```python
from build123d import *

# Parameters (mm, degrees)
ESQUISSE1_R               = 1.25
ESQUISSE1_R_2             = 1.5
ESQUISSE1_W               = 23
ESQUISSE1_H               = 12.5
ESQUISSE1_W_2             = 13
ESQUISSE1_H_2             = 3
ESQUISSE1_W_3             = 3
ESQUISSE1_H_3             = 6
ESQUISSE1_W_4             = 5
ESQUISSE1_W_5             = 5.008466432
ESQUISSE1_W_6             = 3.2
ESQUISSE1_H_4             = 2
T_LE_DE_BASE_PLI_E1_DEPTH = 3
ESQUISSE2_R               = 1.5
ENL_V_MAT_EXTRU_1_DEPTH   = 10


# Sheet-metal steps are written as plain solids
with BuildPart() as part:
    # Esquisse1 → Tôle de base pliée1 (new body)
    with BuildSketch(Plane.XY):
        with BuildLine():
            Line((0, 42.516223037), (0, 2))
            ThreePointArc((0, 2), (0.585786438, 0.585786438), (2, 0))
            Line((2, 0), (58, 0))
            ThreePointArc((58, 0), (59.414213562, 0.585786438), (60, 2))
            Line((60, 2), (60, 40.598160001))
            ThreePointArc((60, 40.598160001), (59.938461819, 41.090466587), (59.757634225, 41.552477522))
            Line((59.757634225, 41.552477522), (54.409971269, 51.401647463))
            ThreePointArc((54.409971269, 51.401647463), (53.538493891, 52.240295654), (52.342948156, 52.423254667))
            Line((52.342948156, 52.423254667), (1.690611112, 44.492147761))
            ThreePointArc((1.690611112, 44.492147761), (0.480332639, 43.816458059), (0, 42.516223037))
        make_face()
        with Locations((51.745273693, 48.75)):
            Circle(ESQUISSE1_R, mode=Mode.SUBTRACT)
        with Locations((20.7, 41.7)):
            Circle(ESQUISSE1_R_2, mode=Mode.SUBTRACT)
        with Locations((4.5, 11)):
            Circle(ESQUISSE1_R_2, mode=Mode.SUBTRACT)
        with Locations((55.5, 11)):
            Circle(ESQUISSE1_R_2, mode=Mode.SUBTRACT)
        with Locations((20.5, 31.75)):
            Rectangle(ESQUISSE1_W, ESQUISSE1_H, mode=Mode.SUBTRACT)
        with Locations((46.2, 6)):
            Rectangle(ESQUISSE1_W_2, ESQUISSE1_H_2, mode=Mode.SUBTRACT)
        with Locations((55.7, 4.5)):
            Rectangle(ESQUISSE1_W_3, ESQUISSE1_H_3, mode=Mode.SUBTRACT)
        with Locations((55.7, 17.5)):
            Rectangle(ESQUISSE1_W_3, ESQUISSE1_H_3, mode=Mode.SUBTRACT)
        with Locations((17.808466432, 6)):
            Rectangle(ESQUISSE1_W_4, ESQUISSE1_H_2, mode=Mode.SUBTRACT)
        with Locations((9.804233216, 6)):
            Rectangle(ESQUISSE1_W_5, ESQUISSE1_H_2, mode=Mode.SUBTRACT)
        with Locations((4.3, 6)):
            Rectangle(ESQUISSE1_W_3, ESQUISSE1_H_2, mode=Mode.SUBTRACT)
        with Locations((4.1, 15.5)):
            Rectangle(ESQUISSE1_W_6, ESQUISSE1_H_4, mode=Mode.SUBTRACT)
        with Locations((4.1, 19)):
            Rectangle(ESQUISSE1_W_6, ESQUISSE1_H_4, mode=Mode.SUBTRACT)
    extrude(amount=-T_LE_DE_BASE_PLI_E1_DEPTH)

    # Esquisse2 → Enlèv. mat.-Extru.1 (cut)
    with BuildSketch(Plane(origin=(0, 0, -3), x_dir=(-1, 0, 0), z_dir=(0, 0, -1))):
        with Locations((-20.66577155, 21.799816522)):
            Circle(ESQUISSE2_R)
    extrude(amount=-ENL_V_MAT_EXTRU_1_DEPTH, mode=Mode.SUBTRACT)


solid = part.part
```
The listing builds one solid part. Answer for the finished solid, in the listing's coordinates (mm). A direction names the side the tool comes from. Round coordinates to 2 decimals unless told otherwise and drop trailing zeros. Loops run counter-clockwise (first coordinate to the right, second up) from the corner with the lowest first, then second, coordinate; pieces in that order, holes last.
1) For faces 1 (the face through (56, 7.5, -1)), 2 (the face through (0.57, 0.6, -1.48)), determine the directions among +Z, -Z, +X, -X, +Y, -Y from which every point of the face is accessible in a straight line to the end or side of a thin tool.
Outcome:
face 1: +Z, -Z
face 2: +Z, -Z, -X, -Y
2) A cutting plane is placed at A-A on x = 29. Determine the outline of the cut face in (y, z).
Outcome:
outline: (0, -3) - (25.5, -3) - (25.5, 0) - (0, 0) - close; (38, -3) - (48.77, -3) - (48.77, 0) - (38, 0) - close
3) For a pull along X with two mould halves and no side action, classify faces 3 (the face through (30, 0, -1)), 4 (the face through (57.2, 17, -1)), 5 (the face through (57.12, 46.41, -1.48)) as released by +X, released by -X, zero draft, split by the parting line, or undercut.
Outcome:
face 3: zero draft
face 4: undercut
face 5: released by +X
4) A cutting plane is placed at C-C on x = 55.5. Determine the outline of the cut face in (y, z).
Outcome:
outline: (0, -3) - (1.5, -3) - (1.5, 0) - (0, 0) - close; (7.5, -3) - (9.5, -3) - (9.5, 0) - (7.5, 0) - close; (12.5, -3) - (14.5, -3) - (14.5, 0) - (12.5, 0) - close; (20.5, -3) - (49.39, -3) - (49.39, 0) - (20.5, 0) - close
5) Consider line 1 (X direction, y = 28, z = -1.25); line 2 (Y direction, x = 52, z = -1.4); line 3 (Y direction, x = 56, z = -1). Determine where each line is inside the solid, lowest interval first.
Outcome:
line 1: x = 0 to 9, 32 to 60
line 2: y = 0 to 4.5, 7.5 to 47.53, 49.97 to 52.37
line 3: y = 0 to 1.5, 7.5 to 9.59, 12.41 to 14.5, 20.5 to 48.47
6) A cutting plane is placed at B-B on y = 22.5. Determine the outline of the cut face in (x, z).
Outcome:
outline: (0, -3) - (19.34, -3) - (19.34, 0) - (0, 0) - close; (21.99, -3) - (60, -3) - (60, 0) - (21.99, 0) - close
7) A cutting plane is placed at D-D on x = 4.5. Determine the outline of the cut face in (y, z).
Outcome:
outline: (0, -3) - (4.5, -3) - (4.5, 0) - (0, 0) - close; (7.5, -3) - (9.5, -3) - (9.5, 0) - (7.5, 0) - close; (12.5, -3) - (14.5, -3) - (14.5, 0) - (12.5, 0) - close; (16.5, -3) - (18, -3) - (18, 0) - (16.5, 0) - close; (20, -3) - (44.93, -3) - (44.93, 0) - (20, 0) - close
8) Given P1, Ø0.9, axis at x = 18.5, z = -2, coming from the +Y side; P2, Ø1.5, axis at x = 55, z = -1.5, coming from the +Y side, each flat-ended and moving along its own axis, determine where each tip first touches the part or whether it passes through.
Outcome:
P1: stops at y = 47.19
P2: stops at y = 51.65
